Geometry check sheet. Reference: drawing and pictorial views, mm from the part's lowest x, y, z. A direction names the side the tool comes from. Coordinates: 2 decimals unless noted, no trailing zeros. Write each loop counter-clockwise with the first axis right and the second up, starting at its lowest first coordinate (ties: lowest second). Pieces come first, ordered by that corner, then holes. Notation, with made-up numbers: (34.25, 72) -> (67.25, 72) arc R27 cw to (67.25, 111) -> close; hole circle Ø1 at (83, 71). An arc over 180 degrees is marked (long way). Use a Markdown table: item, result.
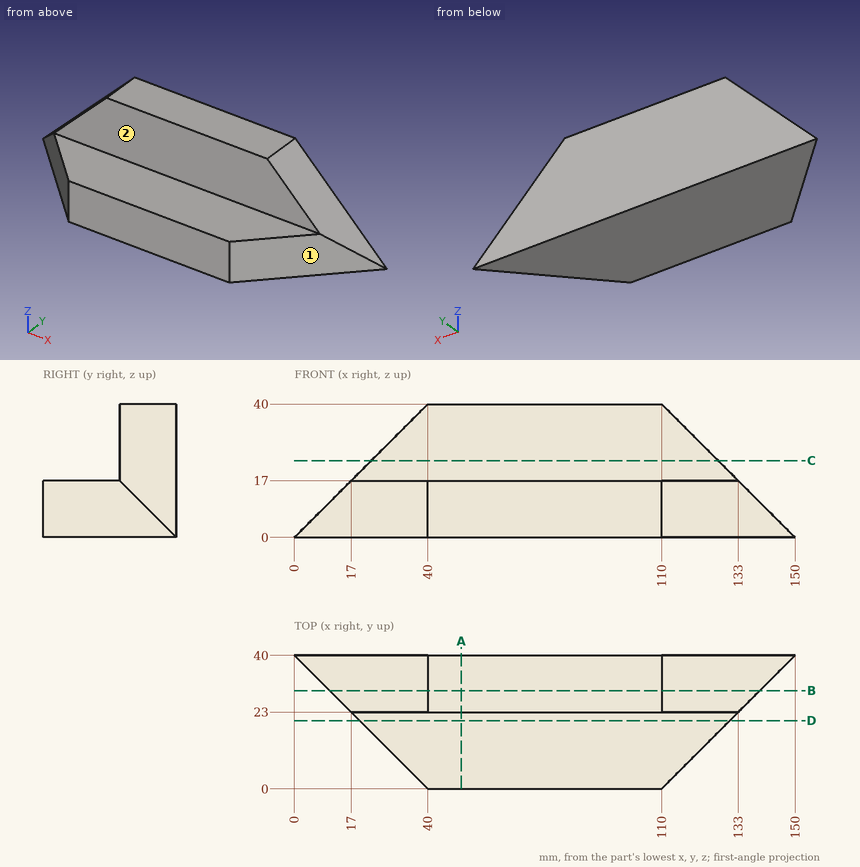
Item 1: Section check C-C on z = 23. Record the boundary of the cut face in (x, y).
Answer block:
| item | result |
|---|---|
| outline | (23, 23) -> (127, 23) -> (127, 40) -> (23, 40) -> close |
Item 2: Section check B-B on y = 29.5. Record the boundary of the cut face in (x, z), then the cut area to 3 significant figures.
Answer block:
| item | result |
|---|---|
| outline | (10.5, 0) -> (139.5, 0) -> (139.5, 10.5) -> (110, 40) -> (40, 40) -> (10.5, 10.5) -> close |
| area | 4,290 mm^2 |
Item 3: Depth check by flat-ended pin: P1, Ø7, axis at x = 76, z = 28, coming from the -Y side; P2, Ø1, axis at y = 19, z = 13.5, coming from the -X side; P3, Ø4, axis at y = 9, z = 5.5, coming from the -X side. Enter the tip coordinate at first touch or a pass-through.
Answer block:
| item | result |
|---|---|
| P1 | stops at y = 23 |
| P2 | stops at x = 20.5 |
| P3 | stops at x = 29 |
Item 4: Section check A-A on x = 50. Record the boundary of the cut face in (y, z).
Answer block:
| item | result |
|---|---|
| outline | (0, 0) -> (40, 0) -> (40, 40) -> (23, 40) -> (23, 17) -> (0, 17) -> close |
Item 5: Section check D-D on y = 20.5. Record the boundary of the cut face in (x, z), then the cut area to 3 significant figures.
Answer block:
| item | result |
|---|---|
| outline | (19.5, 0) -> (130.5, 0) -> (130.5, 17) -> (19.5, 17) -> close |
| area | 1,890 mm^2 |
Item 6: Thickness scan on L1, parallel to Y at x = 35.5, z = 27.5; L2, parallel to Z at x = 20, y = 22; L3, parallel to X at y = 32, z = 8. Record the ranges inside material, lowest first. Write a range as [from, to].
Answer block:
| item | result |
|---|---|
| L1 | y = [23, 40] |
| L2 | z = [0, 17] |
| L3 | x = [8, 142] |
Item 7: Tool access check on the marked faces 1 and 2. Record the directions out of +Z, -Z, +X, -X, +Y, -Y that give a thin tool (end or side, any length) a straight path to the whole face; none if there is none.
Answer block:
| item | result |
|---|---|
| face 1 | +Z, -Z, +X, -Y |
| face 2 | +Z, +X, -X, -Y |
